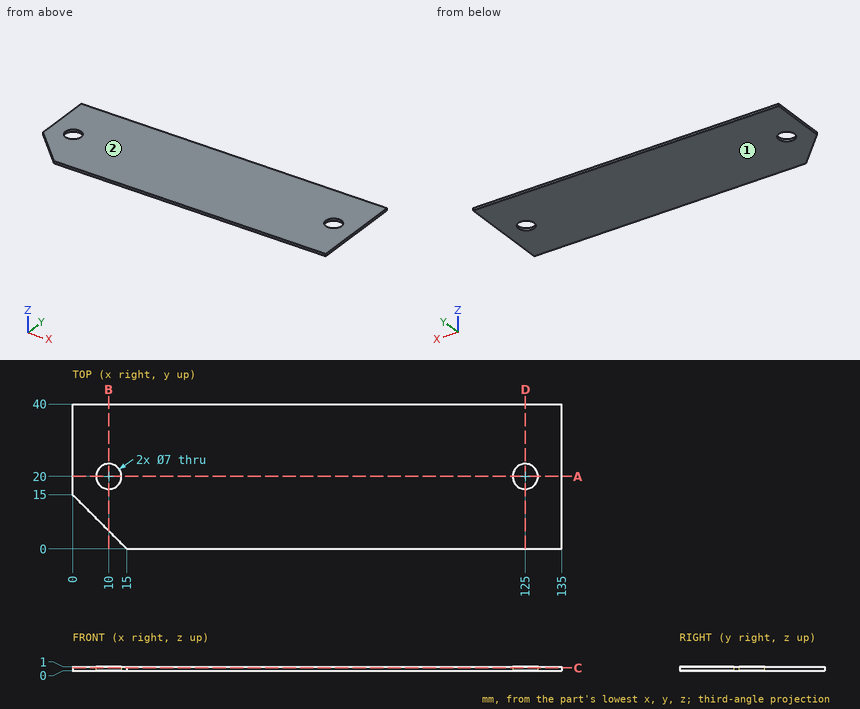
For this review, use the dimensioned drawing (mm, ordinates from the lowest corner) and the shaded views. Give positions to 0.01 mm unless a question says otherwise; leave off trailing zeros. Order: outer loops, then holes, each group sorted by start corner. A loop starts at its lowest first (then second) coordinate and runs counter-clockwise, first axis right, second up. Notation, with made-up numbers: (-24, 32.5) - (29, 32.5) arc R35 cw to (29, 65.5) - close; hole circle Ø8 at (67.25, 24.25). An arc over 180 degrees is marked (long way). Use CSV: the item, a comma, the result in double quotes. Start each with the question number.
Q1. For P1, Ø5.5, axis at x = 125, y = 20, coming from the +Z side, flat-tipped, find the tip position at first contact; note if it passes through.
Q2. Take a section at D-D (x = 125). State the section outline as (y, z) points, and give its area (3 significant figures).
Q3. Take a section at A-A (y = 20). State the section outline as (x, z) points, and give its area (3 significant figures).
Q4. For line 1 (X direction, y = 21.5, z = 0.7); line 2 (Y direction, x = 125, z = 0.5); line 3 (X direction, y = 8.5, z = 0.35), list the stretches that pass through material, from the lowest coordinate up.
Q5. Draft analysis for pull direction Z (two halves, no side actions). For the marked faces 1 and 2, state which applies: pulls with the +Z half, pulls with the -Z half, needs draft (parallel to the pull), parting line crosses it, or undercut.
Q6. Take a section at C-C (z = 0.75). State the section outline as (x, y) points.
Q7. Take a section at B-B (x = 10). State the section outline as (y, z) points, and give its area (3 significant figures).
Calculated:
1,P1,"passes through"
2,outline,"(0, 0) - (16.5, 0) - (16.5, 1) - (0, 1) - close; (23.5, 0) - (40, 0) - (40, 1) - (23.5, 1) - close"
2,area,"33.0 mm²"
3,outline,"(0, 0) - (6.5, 0) - (6.5, 1) - (0, 1) - close; (13.5, 0) - (121.5, 0) - (121.5, 1) - (13.5, 1) - close; (128.5, 0) - (135, 0) - (135, 1) - (128.5, 1) - close"
3,area,"121 mm²"
4,line 1,"x = 0 to 6.84, 13.16 to 121.84, 128.16 to 135"
4,line 2,"y = 0 to 16.5, 23.5 to 40"
4,line 3,"x = 6.5 to 135"
5,face 1,"pulls with the -Z half"
5,face 2,"pulls with the +Z half"
6,outline,"(0, 15) - (15, 0) - (135, 0) - (135, 40) - (0, 40) - close; hole circle Ø7 at (10, 20); hole circle Ø7 at (125, 20)"
7,outline,"(5, 0) - (16.5, 0) - (16.5, 1) - (5, 1) - close; (23.5, 0) - (40, 0) - (40, 1) - (23.5, 1) - close"
7,area,"28.0 mm²"
